from build123d import *

# Parameters (mm, degrees)
ESQUISSE1_W             = 130
ESQUISSE1_H             = 90
BOSS_EXTRU_1_DEPTH      = 2
ESQUISSE2_R             = 1.5
ESQUISSE2_R_2           = 1.25
ESQUISSE2_R_3           = 1
ENL_V_MAT_EXTRU_1_DEPTH = 2
ENL_V_MAT_EXTRU_2_DEPTH = 10
ENL_V_MAT_EXTRU_3_DEPTH = 10
ENL_V_MAT_EXTRU_4_DEPTH = 10


with BuildPart() as part:
    # Esquisse1 → Boss.-Extru.1 (new body)
    with BuildSketch(Plane(origin=(0, 0, 0), x_dir=(1, 0, 0), z_dir=(0, 1, 0))):
        with Locations((-15.798192771, -19.450301205)):
            Rectangle(ESQUISSE1_W, ESQUISSE1_H)
    extrude(amount=BOSS_EXTRU_1_DEPTH)

    # Esquisse2 → Enlèv. mat.-Extru.1 (cut)
    with BuildSketch(Plane(origin=(0, 2, 0), x_dir=(1, 0, 0), z_dir=(0, 1, 0))):
        with Locations(Location((-52.298192771, 12.549698795, 0), (0, 0, 270))):  # turned: the seam where the file's is
            Circle(ESQUISSE2_R)
        with Locations(Location((-7.298192771, 12.549698795, 0), (0, 0, 270))):  # turned: the seam where the file's is
            Circle(ESQUISSE2_R)
        with Locations(Location((-60.798192771, -3.330301205, 0), (0, 0, 270))):  # turned: the seam where the file's is
            Circle(ESQUISSE2_R_2)
        with Locations(Location((-10.798192771, -3.330301205, 0), (0, 0, 270))):  # turned: the seam where the file's is
            Circle(ESQUISSE2_R_2)
        with Locations(Location((-10.798192771, -28.330301205, 0), (0, 0, 270))):  # turned: the seam where the file's is
            Circle(ESQUISSE2_R_2)
        with Locations(Location((-60.798192771, -28.330301205, 0), (0, 0, 270))):  # turned: the seam where the file's is
            Circle(ESQUISSE2_R_2)
        with Locations(Location((-54.868192771, -35.330301205, 0), (0, 0, 270))):  # turned: the seam where the file's is
            Circle(ESQUISSE2_R_3)
        with Locations(Location((-30.968192771, -35.330301205, 0), (0, 0, 270))):  # turned: the seam where the file's is
            Circle(ESQUISSE2_R_3)
        with Locations(Location((-30.968192771, -56.030301205, 0), (0, 0, 270))):  # turned: the seam where the file's is
            Circle(ESQUISSE2_R_3)
        with Locations(Location((-54.868192771, -56.030301205, 0), (0, 0, 270))):  # turned: the seam where the file's is
            Circle(ESQUISSE2_R_3)
        with Locations(Location((-75.798192771, -4.450301205, 0), (0, 0, 270))):  # turned: the seam where the file's is
            Circle(ESQUISSE2_R_2)
        with Locations(Location((-75.798192771, -59.450301205, 0), (0, 0, 270))):  # turned: the seam where the file's is
            Circle(ESQUISSE2_R_2)
        with Locations(Location((44.201807229, 20.549698795, 0), (0, 0, 270))):  # turned: the seam where the file's is
            Circle(ESQUISSE2_R_2)
        with Locations(Location((44.201807229, -59.450301205, 0), (0, 0, 270))):  # turned: the seam where the file's is
            Circle(ESQUISSE2_R_2)
        with Locations(Location((-75.798192771, 20.549698795, 0), (0, 0, 270))):  # turned: the seam where the file's is
            Circle(ESQUISSE2_R_2)
    extrude(amount=-ENL_V_MAT_EXTRU_1_DEPTH, mode=Mode.SUBTRACT)

    # Esquisse3 → Enlèv. mat.-Extru.2 (cut)
    with BuildSketch(Plane(origin=(0, 2, 0), x_dir=(1, 0, 0), z_dir=(0, 1, 0))):
        Polygon((39.201807229, 20.549698795), (-1.521135019, 20.549698795), (-2.521135019, 19.549698795), (-2.521135019, 9.549698795), (-3.521135019, 8.549698795), (-6.521135019, 8.549698795), (-7.521135019, 7.549698795), (-7.521135019, -30.450301205), (-8.521135019, -31.450301205), (-26.521135019, -31.450301205), (-27.521135019, -32.450301205), (-27.521135019, -58.450301205), (-26.521135019, -59.450301205), (39.201807229, -59.450301205), (39.201807229, -56.450301205), (41.201807229, -54.450301205), (44.201807229, -54.450301205), (44.201807229, 15.549698795), (41.201807229, 15.549698795), (39.201807229, 17.549698795), align=None)
    extrude(amount=-ENL_V_MAT_EXTRU_2_DEPTH, mode=Mode.SUBTRACT)

    # Esquisse4 → Enlèv. mat.-Extru.3 (cut)
    with BuildSketch(Plane(origin=(0, 2, 0), x_dir=(1, 0, 0), z_dir=(0, 1, 0))):
        Polygon((-58.798192771, -6.330301205), (-57.798192771, -5.330301205), (-13.798192771, -5.330301205), (-12.798192771, -6.330301205), (-12.798192771, -25.330301205), (-13.798192771, -26.330301205), (-57.798192771, -26.330301205), (-58.798192771, -25.330301205), align=None)
    extrude(amount=-ENL_V_MAT_EXTRU_3_DEPTH, mode=Mode.SUBTRACT)

    # Esquisse5 → Enlèv. mat.-Extru.4 (cut)
    with BuildSketch(Plane(origin=(0, 2, 0), x_dir=(1, 0, 0), z_dir=(0, 1, 0))):
        Polygon((-46.298192771, 20.549698795), (-13.298192771, 20.549698795), (-12.298192771, 19.549698795), (-12.298192771, 1.549698795), (-13.298192771, 0.549698795), (-46.298192771, 0.549698795), (-47.298192771, 1.549698795), (-47.298192771, 19.549698795), align=None)
    extrude(amount=-ENL_V_MAT_EXTRU_4_DEPTH, mode=Mode.SUBTRACT)


solid = part.part
Model file for the job. Use its own axes, mm. Coordinates: 2 decimals unless noted, no trailing zeros. Write each loop counter-clockwise with the first axis right and the second up, starting at its lowest first coordinate (ties: lowest second). Pieces come first, ordered by that corner, then holes. Notation, with made-up numbers: (67, 21.25) -> (77, 21.25) arc R22 ccw to (77, 45.25) -> close; hole circle Ø8 at (73, 67). An arc over 180 degrees is marked (long way). One line per item, written item: value. Start each with the question number.
1) Slice it at D-D on z = 43.5. Write the cut outline in (x, y), then the cut area to 3 significant figures.
2) Slice it at C-C on x = -17. Write the cut outline in (y, z), then the cut area to 3 significant figures.
3) Pull direction X, two halves, no side cores. Call faces 1 (the face through (-9.56, 1.01, 3.17)), 2 (the face through (-46, 2, 29)): +X half, -X half, draft (parallel to the pull), parting line (faces both ways), or undercut.
4) Slice it at A-A on x = -45. Write the cut outline in (y, z).
5) Flat gauge pin, fed straight in: pin 1 Ø2 at (x, z) = (-10.8, 28.33) entering from +Y. Where does the tip first touch, or does it go through?
6) Slice it at B-B on z = -4.5. Write the cut outline in (x, y).
7) Probe probe 1 along X at (y, z) = (1.1, -2.5); probe 2 along X at (y, z) = (1.6, -15); probe 3 along Z at (x, y) = (20.5, 1.55). List the from-to ranges inside material, lowest first.
Answers follow:
1. outline: (-80.8, 0) -> (-27.52, 0) -> (-27.52, 2) -> (-80.8, 2) -> close; (44.2, 0) -> (49.2, 0) -> (49.2, 2) -> (44.2, 2) -> close
1. area: 117 mm2
2. outline: (0, -25.55) -> (2, -25.55) -> (2, -20.55) -> (0, -20.55) -> close; (0, -0.55) -> (2, -0.55) -> (2, 5.33) -> (0, 5.33) -> close; (0, 26.33) -> (2, 26.33) -> (2, 31.45) -> (0, 31.45) -> close; (0, 59.45) -> (2, 59.45) -> (2, 64.45) -> (0, 64.45) -> close
2. area: 42.0 mm2
3. face 1: undercut
3. face 2: draft
4. outline: (0, -25.55) -> (2, -25.55) -> (2, -20.55) -> (0, -20.55) -> close; (0, -0.55) -> (2, -0.55) -> (2, 5.33) -> (0, 5.33) -> close; (0, 26.33) -> (2, 26.33) -> (2, 64.45) -> (0, 64.45) -> close
5. pin 1: through
6. outline: (-80.8, 0) -> (-47.3, 0) -> (-47.3, 2) -> (-80.8, 2) -> close; (-12.3, 0) -> (-7.52, 0) -> (-7.52, 2) -> (-12.3, 2) -> close; (44.2, 0) -> (49.2, 0) -> (49.2, 2) -> (44.2, 2) -> close
7. probe 1: -80.8 to -47.3, -12.3 to -7.52, 44.2 to 49.2
7. probe 2: -80.8 to -47.3, -12.3 to -2.52, 44.2 to 49.2
7. probe 3: -25.55 to -20.55, 59.45 to 64.45
